```python
from build123d import *

# Parameters (mm, degrees)
F0_W     = 120
F0_H     = 60
F3_DEPTH = 5
F1_W     = 75
F1_H     = 30
F4_DEPTH = 1
F2_W     = 70
F2_H     = 26
F5_DEPTH = 10


with BuildPart() as f3:
    # F0 (on Top) → F3 (new body)
    with BuildSketch(Plane.XY):
        Rectangle(F0_W, F0_H)
    extrude(amount=-F3_DEPTH)

    # F1 (on Top) → F4 (cut)
    with BuildSketch(Plane.XY):
        Rectangle(F1_W, F1_H)
    extrude(amount=-F4_DEPTH, mode=Mode.SUBTRACT)

    # F2 (on Top) → F5 (cut)
    with BuildSketch(Plane.XY):
        Rectangle(F2_W, F2_H)
    extrude(amount=-F5_DEPTH, mode=Mode.SUBTRACT)


solid = f3.part
```
Geometry: final body of the model. Coordinates: model frame, mm. A direction names the side the tool comes from. Round coordinates to 2 decimals unless told otherwise and drop trailing zeros. Write each loop counter-clockwise with the first axis right and the second up, starting at its lowest first coordinate (ties: lowest second). Pieces come first, ordered by that corner, then holes. Notation, with made-up numbers: M -17.5,82.5 L 14.5,82.5 A36 ccw 14.5,121.5 Z; hole C 89.25,85.5 d8. An arc over 180 degrees is marked long. Answer in a Markdown table with one row per item. Add a question column.
(1) Draft query along X for faces 3 (the face through (-3, -13.3, -1)), 4 (the face through (-1, 30, -2)), 5 (the face through (60, 0, -2)). Return one class per face: pulls with the +X half, pulls with the -X half, needs draft (parallel to the pull), parting line crosses it, or undercut.
(2) Cut plane C-C, the plane z = -2.4. Return the cut outline in (x, y), then the cut area to 3 significant figures.
(3) Reachability of faces 1 (the face through (35, 0, -3)), 2 (the face through (-1, 14, -5)) from +Z, -Z, +X, -X, +Y, -Y: full face, straight path, thin tool, end or side. Return the list, or none.
(4) Cut plane B-B, the plane y = -4. Return the cut outline in (x, z).
(5) Ray query, L1, parallel to X at y = -4.5, z = -1.4; L2, parallel to Y at x = 23, z = -0.5; L3, parallel to Y at x = 7, z = -4.1. Return the intervals inside material, ascending.
(6) Cut plane A-A, the plane x = 4. Return the cut outline in (y, z), then the cut area to 3 significant figures.
Established:
| question | item | result |
|---|---|---|
| 1 | face 3 | undercut |
| 1 | face 4 | needs draft |
| 1 | face 5 | pulls with the +X half |
| 2 | outline | M -60,-30 L 60,-30 L 60,30 L -60,30 Z; hole M -35,-13 L 35,-13 L 35,13 L -35,13 Z |
| 2 | area | 5,380 mm² |
| 3 | face 1 | +Z, -Z |
| 3 | face 2 | -Z, +X, -X, +Y, -Y |
| 4 | outline | M -60,-5 L -35,-5 L -35,-1 L -37.5,-1 L -37.5,0 L -60,0 Z; M 35,-5 L 60,-5 L 60,0 L 37.5,0 L 37.5,-1 L 35,-1 Z |
| 5 | L1 | -60 to -35, 35 to 60 |
| 5 | L2 | -30 to -15, 15 to 30 |
| 5 | L3 | -30 to -13, 13 to 30 |
| 6 | outline | M -30,-5 L -13,-5 L -13,-1 L -15,-1 L -15,0 L -30,0 Z; M 13,-5 L 30,-5 L 30,0 L 15,0 L 15,-1 L 13,-1 Z |
| 6 | area | 166 mm² |
